Study the drawing (mm; zero at the part's minimum x, y, z) and answer. Give positions to 0.01 mm unless a question says otherwise; leave off trailing zeros. Write each loop counter-clockwise with the first axis right and the second up, starting at its lowest first coordinate (ties: lowest second). Pieces come first, ordered by that corner, then holes. Notation, with made-up numbers: (81, 2) -> (102, 2) arc R18 cw to (102, 35) -> close; hole circle Ø10 at (86, 79). An arc over 180 degrees is marked (long way). Use CSV: the item, a comma, the result in double quotes. Start each with the question number.
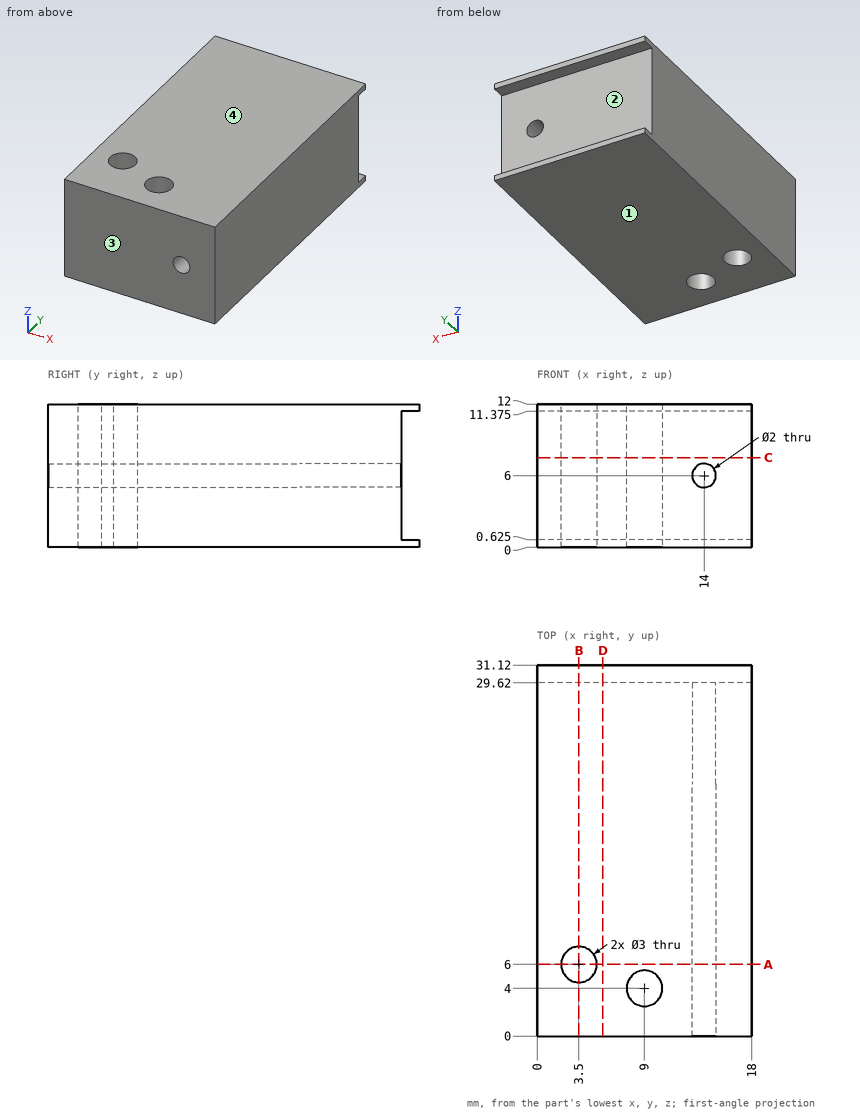
Q1. Straight lines are drawn through the part: L1, parallel to Z at x = 14, y = 27; L2, parallel to Z at x = 11.5, y = 30 (3 decimals); L3, parallel to Y at x = 9, z = 3.25. For each, find the intervals that lie inside material, in ascending order.
Q2. Section B-B on x = 3.5 is taken. Give the vertices of the cut face in (y, z) (3 decimals), then the cut area to 3 significant figures.
Q3. The mould has two halves that part along Z. Classify the marked faces 1, 2, 3 and 4: +Z half, -Z half, draft (parallel to the pull), parting line (faces both ways), or undercut.
Q4. Section D-D on x = 5.5 is taken. Give the vertices of the cut face in (y, z) (3 decimals), then the cut area to 3 significant figures.
Q5. Flat-ended cylindrical pins translate along their axes: pin 1 Ø4 at (x, z) = (9.5, 6) entering from -Y; pin 2 Ø2.5 at (x, z) = (14, 6) entering from +Y. Find the tip coordinate at first contact, or state that the pin passes through.
Q6. Section A-A on y = 6 is taken. Give the vertices of the cut face in (x, z).
Q7. Section C-C on z = 7.5 is taken. Give the vertices of the cut face in (x, y), then the cut area to 3 significant figures.
Output:
1,L1,"0 to 5, 7 to 12"
1,L2,"0 to 0.625, 11.375 to 12"
1,L3,"0 to 2.5, 5.5 to 29.62"
2,outline,"(0, 0) -> (4.5, 0) -> (4.5, 12) -> (0, 12) -> close; (7.5, 0) -> (31.12, 0) -> (31.12, 0.625) -> (29.62, 0.625) -> (29.62, 11.375) -> (31.12, 11.375) -> (31.12, 12) -> (7.5, 12) -> close"
2,area,"321 mm²"
3,face 1,"-Z half"
3,face 2,"undercut"
3,face 3,"draft"
3,face 4,"+Z half"
4,outline,"(0, 0) -> (31.12, 0) -> (31.12, 0.625) -> (29.62, 0.625) -> (29.62, 11.375) -> (31.12, 11.375) -> (31.12, 12) -> (0, 12) -> close"
4,area,"357 mm²"
5,pin 1,"y = 0"
5,pin 2,"y = 29.62"
6,outline,"(0, 0) -> (2, 0) -> (2, 12) -> (0, 12) -> close; (5, 0) -> (18, 0) -> (18, 12) -> (5, 12) -> close; hole circle Ø2 at (14, 6)"
7,outline,"(0, 0) -> (18, 0) -> (18, 29.62) -> (0, 29.62) -> close; hole circle Ø3 at (3.5, 6); hole circle Ø3 at (9, 4)"
7,area,"519 mm²"
